Design review of the part built by this model. Coordinates are the model's own, in mm. A direction names the side the tool comes from. Coordinates: 2 decimals unless noted, no trailing zeros. Loops run counter-clockwise (first coordinate to the right, second up) from the corner with the lowest first, then second, coordinate; pieces in that order, holes last.
Q1. Draft analysis for pull direction Z (two halves, no side actions). For faces 1 (the face through (28.194, 2, -10)), 2 (the face through (24, 10.795, -10)), 3 (the face through (-2.129, 9.69, -6.633)), state which applies: released by +Z, released by -Z, zero draft, split by the parting line, or undercut.
Q2. For P1, Ø1.8, axis at x = 23.5, y = 8.5, coming from the +Z side; P2, Ø5, axis at y = 18.5, z = -10, coming from the -X side; P3, Ø3.5, axis at x = 26, z = -9.5, coming from the +Y side, all flat-tipped, find the tip position at first contact; note any pin that passes through.
Q3. Machinability: for faces 4 (the face through (11, 7, 0)), 5 (the face through (11, 7, -20.32)), 6 (the face through (24, 7, -7.302)), which of the approach directions +Z, -Z, +X, -X, +Y, -Y give a long, thin tool a straight path to every point of the face, cutting with its end or side? Answer none if there is none.
Q4. Add section C-C on x = -21. Give the boundary of the cut face in (y, z) (3 decimals), and give its area (3 significant figures).
Q5. Add section A-A on z = -23. Give the boundary of the cut face in (x, y), and give its area (3 significant figures).
Q6. Wall thickness on probe 1 along Y at (x, z) = (1, -8); probe 2 along X at (y, z) = (3.5, -4.5); probe 3 along X at (y, z) = (4.25, -24): over which ranges is each line inside the solid? List them lowest first.
Q7. Add section D-D on z = 3. Give the boundary of the cut face in (x, y).
```python
from build123d import *
from OCP.BRepFilletAPI import BRepFilletAPI_MakeChamfer

# Parameters (mm, degrees)
BOSS_EXTRUDE1_DEPTH    = 13.97
SKETCH2_W              = 12.192
SKETCH2_H              = 10.668
BOSS_EXTRUDE2_DEPTH    = 3.175
SKETCH3_W              = 5.715
SKETCH3_H              = 3.175
CUT_EXTRUDE1_DEPTH     = 7.62
CHAMFER1_SIZE          = 1.016
CHAMFER1_SIZE2         = 0.586587873
CUT_EXTRUDE2_START     = -5.207
CUT_EXTRUDE2_OUTLINE_R = 1.905
CUT_EXTRUDE2_DEPTH     = 5.207
FILLET1_R              = 2.54
SKETCH5_R              = 4.445
BOSS_EXTRUDE3_DEPTH    = 4.318
SKETCH6_R              = 1.905


# Read off the part's stored shape, not the designer's step: Cut-Extrude2
with BuildPart() as part:
    # Sketch1 → Boss-Extrude1 (new body)
    with BuildSketch(Plane(origin=(0, 0, 0), x_dir=(1, 0, 0), z_dir=(0, 1, 0))):
        Polygon((0, 0), (0, 20.32), (19.812, 20.32), (19.812, 27.432), (25.019, 27.432), (25.019, -7.112), (19.812, -7.112), (19.812, 0), align=None)
    extrude(amount=BOSS_EXTRUDE1_DEPTH)

    # Sketch2 → Boss-Extrude2 (add)
    with BuildSketch(Plane(origin=(25.019, 0, 0), x_dir=(0, 0, -1), z_dir=(1, 0, 0))):
        with Locations((10.16, 6.985)):
            Rectangle(SKETCH2_W, SKETCH2_H)
    extrude(amount=BOSS_EXTRUDE2_DEPTH)

    # Sketch3 → Cut-Extrude1 (cut)
    with BuildSketch(Plane(origin=(28.194, 0, 0), x_dir=(0, 0, -1), z_dir=(1, 0, 0))):
        Polygon((5.715, 10.795), (14.605, 10.795), (14.605, 4.7625), (13.0175, 3.175), (7.3025, 3.175), (5.715, 4.7625), align=None)
        with Locations((10.16, 6.985)):
            Rectangle(SKETCH3_W, SKETCH3_H, mode=Mode.SUBTRACT)
    extrude(amount=-CUT_EXTRUDE1_DEPTH, mode=Mode.SUBTRACT)

    # Chamfer1: one chamfer whose edges measure the first distance from different faces: ONE call of the kernel's chamfer builder (chamfer() names one face for all edges)
    chamfer1_edges_1 = [part.edges().sort_by_distance(p)[0] for p in [
        (28.194, 6.985, -7.3025),
    ]]
    chamfer1_side_1 = [part.faces().sort_by_distance(p)[0] for p in [
        (24.384, 6.985, -7.3025),
    ]]
    chamfer1_edges_2 = [part.edges().sort_by_distance(p)[0] for p in [
        (28.194, 8.5725, -10.16),
    ]]
    chamfer1_side_2 = [part.faces().sort_by_distance(p)[0] for p in [
        (24.384, 8.5725, -10.16),
    ]]
    chamfer1_edges_3 = [part.edges().sort_by_distance(p)[0] for p in [
        (28.194, 6.985, -13.0175),
    ]]
    chamfer1_side_3 = [part.faces().sort_by_distance(p)[0] for p in [
        (24.384, 6.985, -13.0175),
    ]]
    chamfer1_edges_4 = [part.edges().sort_by_distance(p)[0] for p in [
        (28.194, 5.3975, -10.16),
    ]]
    chamfer1_side_4 = [part.faces().sort_by_distance(p)[0] for p in [
        (24.384, 5.3975, -10.16),
    ]]
    chamfer1 = BRepFilletAPI_MakeChamfer(part.part.solid().wrapped)
    for e in chamfer1_edges_1:
        chamfer1.Add(CHAMFER1_SIZE, CHAMFER1_SIZE2, e.wrapped, chamfer1_side_1[0].wrapped)  # the first distance lies on this face
    for e in chamfer1_edges_2:
        chamfer1.Add(CHAMFER1_SIZE, CHAMFER1_SIZE2, e.wrapped, chamfer1_side_2[0].wrapped)  # the first distance lies on this face
    for e in chamfer1_edges_3:
        chamfer1.Add(CHAMFER1_SIZE, CHAMFER1_SIZE2, e.wrapped, chamfer1_side_3[0].wrapped)  # the first distance lies on this face
    for e in chamfer1_edges_4:
        chamfer1.Add(CHAMFER1_SIZE, CHAMFER1_SIZE2, e.wrapped, chamfer1_side_4[0].wrapped)  # the first distance lies on this face
    add(Compound.cast(chamfer1.Shape()), mode=Mode.REPLACE)

    # Cut-Extrude2 outline → Cut-Extrude2 (cut)
    with BuildSketch(Plane(origin=(25.019, 0, 0), x_dir=(0, 0, -1), z_dir=(1, 0, 0)).offset(CUT_EXTRUDE2_START)):
        with BuildLine():
            ThreePointArc((27.432, 6.985), (25.386140867, 2.045859133), (20.447, 0))
            Line((20.447, 0), (27.432, 0))
            Line((27.432, 0), (27.432, 6.985))
        make_face()
        with BuildLine():
            ThreePointArc((20.447, 13.97), (25.386140867, 11.924140867), (27.432, 6.985))
            Line((27.432, 6.985), (27.432, 13.97))
            Line((27.432, 13.97), (20.447, 13.97))
        make_face()
        with BuildLine():
            Line((-7.112, 0), (-0.127, 0))
            ThreePointArc((-0.127, 0), (-5.066140867, 2.045859133), (-7.112, 6.985))
            Line((-7.112, 6.985), (-7.112, 0))
        make_face()
        with BuildLine():
            Line((-7.112, 13.97), (-7.112, 6.985))
            ThreePointArc((-7.112, 6.985), (-5.066140867, 11.924140867), (-0.127, 13.97))
            Line((-0.127, 13.97), (-7.112, 13.97))
        make_face()
        with Locations((23.622, 6.985)):
            Circle(CUT_EXTRUDE2_OUTLINE_R)
        with Locations((-3.302, 6.985)):
            Circle(CUT_EXTRUDE2_OUTLINE_R)
    extrude(amount=CUT_EXTRUDE2_DEPTH, mode=Mode.SUBTRACT)

    # Fillet1
    fillet1_edges = [part.edges().sort_by_distance(p)[0] for p in [
        (0, 6.985, 0),
        (0, 6.985, -20.32),
    ]]
    fillet(fillet1_edges, radius=FILLET1_R)

    # Sketch5 → Boss-Extrude3 (add)
    with BuildSketch(Plane.ZY):
        with Locations(Location((-10.16, 6.985, 0), (0, 0, 180))):
            Circle(SKETCH5_R)
    extrude(amount=BOSS_EXTRUDE3_DEPTH)

    # Sweep1: sweep along a path in Sketch7
    with BuildLine(Plane(origin=(0, 0, -10.16), x_dir=(-1, 0, 0), z_dir=(0, 0, -1))) as sweep1_path:
        Line((4.318, 6.985), (29.718, 6.985))
        ThreePointArc((29.718, 6.985), (36.836393375, 17.323984324), (24.638, 20.284612663))
    # Sketch6 → Sweep1 (sweep)
    with BuildSketch(Plane.ZY.offset(4.318)):
        with Locations((-10.16, 6.985)):
            Circle(SKETCH6_R)
    sweep(path=sweep1_path.line)


solid = part.part
```
Entries:
1. face 1: zero draft
1. face 2: undercut
1. face 3: split by the parting line
2. P1: stops at z = 7.08
2. P2: stops at x = -39.14
2. P3: stops at y = 13.97
3. face 4: +Z, -X, +Y, -Y
3. face 5: -Z, -X, +Y, -Y
3. face 6: +X
4. outline: circle Ø3.81 at (6.985, -10.16)
4. area: 11.4 mm2
5. outline: (19.81, 0.48) - (25.02, 0.48) - (25.02, 5.18) - (19.81, 5.18) - close; (19.81, 8.79) - (25.02, 8.79) - (25.02, 13.49) - (19.81, 13.49) - close
5. area: 49.0 mm2
6. probe 1: y = 0 to 13.97
6. probe 2: x = 0 to 28.19
6. probe 3: x = 19.81 to 25.02
7. outline: (19.81, 0.62) - (25.02, 0.62) - (25.02, 5.1) - (19.81, 5.1) - close; (19.81, 8.87) - (25.02, 8.87) - (25.02, 13.35) - (19.81, 13.35) - close
